from build123d import *

# Parameters (mm, degrees)
F0_W      = 86
F0_H      = 45
F1_DEPTH  = 3
F2_R      = 1.35
F2_W      = 68
F2_H      = 41
F3_DEPTH  = 22
F4_R      = 1.4
F5_DEPTH  = 6
F7_DEPTH  = 3.001
F8_R      = 3
F9_W      = 2
F9_H      = 28
F9_H_2    = 8
F10_DEPTH = 2.5


with BuildPart() as f1:
    # F0 (on Top) → F1 (new body)
    with BuildSketch(Plane.XY):
        Rectangle(F0_W, F0_H)
    extrude(amount=F1_DEPTH)

    # F2 (on face) → F3 (join)
    with BuildSketch(Plane.XY.offset(3)):
        Polygon((43, 22.5), (-43, 22.5), (-43, 14.5), (-36, 14.5), (-36, -14.5), (-43, -14.5), (-43, -22.5), (43, -22.5), (43, -14.5), (36, -14.5), (36, 14.5), (43, 14.5), align=None)
        with Locations((-39, -18.5)):
            Circle(F2_R, mode=Mode.SUBTRACT)
        with Locations((39, -18.5)):
            Circle(F2_R, mode=Mode.SUBTRACT)
        with Locations((-39, 18.5)):
            Circle(F2_R, mode=Mode.SUBTRACT)
        Rectangle(F2_W, F2_H, mode=Mode.SUBTRACT)
        with Locations((39, 18.5)):
            Circle(F2_R, mode=Mode.SUBTRACT)
    extrude(amount=F3_DEPTH)

    # F4 (on face) → F5 (join)
    with BuildSketch(Plane.XY.offset(3)):
        with BuildLine():
            Line((-28.9413119942, 15.2550414599), (-29.2586880058, 15.2550414599))
            ThreePointArc((-29.2586880058, 15.2550414599), (-29.1, 15.25), (-28.9413119942, 15.2550414599))
        make_face()
        with BuildLine():
            Line((-34, 15.2550414599), (-29.2586880058, 15.2550414599))
            Line((-29.2586880058, 15.2550414599), (-28.9413119942, 15.2550414599))
            ThreePointArc((-28.9413119942, 15.2550414599), (-27.3470376902, 15.9675513639), (-26.6080353575, 17.5497196457))
            Line((-26.6080353575, 17.5497196457), (-26.6080353575, 17.9502803543))
            Line((-26.6080353575, 17.9502803543), (-26.6080353575, 20.5))
            Line((-26.6080353575, 20.5), (-34, 20.5))
            Line((-34, 20.5), (-34, 15.2550414599))
        make_face()
        with Locations((-29.1, 17.75)):
            Circle(F4_R, mode=Mode.SUBTRACT)
        with BuildLine():
            Line((-26.6080353575, 17.9502803543), (-26.6080353575, 17.5497196457))
            ThreePointArc((-26.6080353575, 17.5497196457), (-26.6, 17.75), (-26.6080353575, 17.9502803543))
        make_face()
        with BuildLine():
            Line((-26.5361216883, -20.5), (-26.6006603156, -17.6925444326))
            ThreePointArc((-26.6006603156, -17.6925444326), (-27.2968273142, -16.018362548), (-28.9414728026, -15.2550312371))
            Line((-28.9414728026, -15.2550312371), (-29.2585271974, -15.2550312371))
            Line((-29.2585271974, -15.2550312371), (-34, -15.2550312371))
            Line((-34, -15.2550312371), (-34, -20.5))
            Line((-34, -20.5), (-26.5361216883, -20.5))
        make_face()
        with Locations((-29.1, -17.75)):
            Circle(F4_R, mode=Mode.SUBTRACT)
        with BuildLine():
            Line((-29.2585271974, -15.2550312371), (-28.9414728026, -15.2550312371))
            ThreePointArc((-28.9414728026, -15.2550312371), (-29.1, -15.25), (-29.2585271974, -15.2550312371))
        make_face()
        with BuildLine():
            Line((26.6080353575, 17.5497196457), (26.6080353575, 17.9502803543))
            ThreePointArc((26.6080353575, 17.9502803543), (26.6, 17.75), (26.6080353575, 17.5497196457))
        make_face()
        with BuildLine():
            Line((26.6080353575, 20.5), (26.6080353575, 17.9502803543))
            Line((26.6080353575, 17.9502803543), (26.6080353575, 17.5497196457))
            ThreePointArc((26.6080353575, 17.5497196457), (27.4045208473, 15.9127873169), (29.1, 15.25))
            ThreePointArc((29.1, 15.25), (29.1012864239, 15.250000331), (29.1025728475, 15.2500013239))
            Line((29.1025728475, 15.2500013239), (34, 15.2550414599))
            Line((34, 15.2550414599), (34, 20.5))
            Line((34, 20.5), (26.6080353575, 20.5))
        make_face()
        with Locations((29.1, 17.75)):
            Circle(F4_R, mode=Mode.SUBTRACT)
        with BuildLine():
            Line((28.9479452437, -15.2546284142), (29.2524526886, -15.254652694))
            ThreePointArc((29.2524526886, -15.254652694), (29.1001993362, -15.2500000079), (28.9479452437, -15.2546284142))
        make_face()
        with BuildLine():
            Line((34, -15.2550312371), (29.2524526886, -15.254652694))
            Line((29.2524526886, -15.254652694), (28.9479452437, -15.2546284142))
            ThreePointArc((28.9479452437, -15.2546284142), (27.236154388, -16.0838428842), (26.6032541645, -17.8775156186))
            Line((26.6032541645, -17.8775156186), (26.7371915935, -20.5))
            Line((26.7371915935, -20.5), (34, -20.5))
            Line((34, -20.5), (34, -15.2550312371))
        make_face()
        with Locations((29.1, -17.75)):
            Circle(F4_R, mode=Mode.SUBTRACT)
    extrude(amount=F5_DEPTH)

    # F6 (on face) → F7 (cut, through all)
    with BuildSketch(Plane.XY.offset(3)):
        with BuildLine():
            Line((-43, 8.25), (-40, 8.25))
            ThreePointArc((-40, 8.25), (-38.25, 10), (-40, 11.75))
            Line((-40, 11.75), (-43, 11.75))
            Line((-43, 11.75), (-43, 8.25))
        make_face()
        with BuildLine():
            Line((-43, -11.75), (-40, -11.75))
            ThreePointArc((-40, -11.75), (-38.25, -10), (-40, -8.25))
            Line((-40, -8.25), (-43, -8.25))
            Line((-43, -8.25), (-43, -11.75))
        make_face()
        with BuildLine():
            ThreePointArc((40, 11.75), (38.25, 10), (40, 8.25))
            Line((40, 8.25), (43, 8.25))
            Line((43, 8.25), (43, 11.75))
            Line((43, 11.75), (40, 11.75))
        make_face()
        with BuildLine():
            ThreePointArc((40, -8.25), (38.25, -10), (40, -11.75))
            Line((40, -11.75), (43, -11.75))
            Line((43, -11.75), (43, -8.25))
            Line((43, -8.25), (40, -8.25))
        make_face()
    extrude(amount=-F7_DEPTH, mode=Mode.SUBTRACT)

    # F8
    f8_edges = [f1.edges().sort_by_distance(p)[0] for p in [
        (-43, -22.5, 12.5),
        (-43, 14.5, 14),
        (-43, 22.5, 12.5),
        (-43, -14.5, 14),
        (43, -22.5, 12.5),
        (43, -14.5, 14),
        (43, 14.5, 14),
        (43, 22.5, 12.5),
    ]]
    fillet(f8_edges, radius=F8_R)

    # F9 (on face) → F10 (cut)
    with BuildSketch(Plane.XY.offset(25)):
        with Locations((-35, 0)):
            Rectangle(F9_W, F9_H)
        with Locations((35, -9.5)):
            Rectangle(F9_W, F9_H_2)
    extrude(amount=-F10_DEPTH, mode=Mode.SUBTRACT)


solid = f1.part
Work out the finished part from the listing and answer in its coordinate system (mm). A direction names the side the tool comes from. Give positions to 0.01 mm unless a question says otherwise; leave off trailing zeros. Write each loop counter-clockwise with the first axis right and the second up, starting at its lowest first coordinate (ties: lowest second). Pieces come first, ordered by that corner, then holes.
Q1. The part is cut by section C-C on y = 10. Give the vertices of the cut face in (x, z).
Answer:
outline: (-38.25, 0) - (38.25, 0) - (38.25, 3) - (36, 3) - (36, 25) - (34, 25) - (34, 3) - (-34, 3) - (-34, 22.5) - (-36, 22.5) - (-36, 3) - (-38.25, 3) - close
Q2. A tool of negligible diameter and unlimited length cuts with its end or side. For faces 5 (the face through (38, -14.5, 14)), 6 (the face through (35, -5.5, 24)), 7 (the face through (-39.29, 17.18, 13.85)), from which of +Z, -Z, +X, -X, +Y, -Y can it reach the whole face along a straight path? Write none if from no direction.
Answer:
face 5: +Z, +X
face 6: +Z, +X, -X
face 7: +Z
Q3. The part is cut by section A-A on z = 23.75. State how many separate pieces and enclosed holes the cut face has, and give its area (3 significant figures).
Answer:
separate pieces: 2
enclosed holes: 4
area: 566 mm2
Q4. Straight lines are drawn through the part: L1, parallel to Y at x = -29, z = 6.5; L2, parallel to Y at x = 39, z = 8.25; L3, parallel to Y at x = 9, z = 22. For each, find the intervals that lie inside material, in ascending order.
Answer:
L1: y = -22.5 to -19.15, -16.35 to -15.25, 15.25 to 16.35, 19.15 to 22.5
L2: y = -22.5 to -19.85, -17.15 to -14.5, 14.5 to 17.15, 19.85 to 22.5
L3: y = -22.5 to -20.5, 20.5 to 22.5
Q5. The part is cut by section D-D on y = -3. Give the vertices of the cut face in (x, z).
Answer:
outline: (-43, 0) - (43, 0) - (43, 3) - (36, 3) - (36, 25) - (34, 25) - (34, 3) - (-34, 3) - (-34, 22.5) - (-36, 22.5) - (-36, 3) - (-43, 3) - close
Q6. The part is cut by section B-B on x = -19. Give the vertices of the cut face in (y, z).
Answer:
outline: (-22.5, 0) - (22.5, 0) - (22.5, 25) - (20.5, 25) - (20.5, 3) - (-20.5, 3) - (-20.5, 25) - (-22.5, 25) - close
Q7. Given pin 1 (2 mm diameter, centred on y = 3, z = 9, fed in from +X); pin 2 (6.5 mm diameter, centred on y = 6, z = 14.5, fed in from -X); pin 3 (2 mm diameter, centred on x = -6.5, y = -11, fed in from +Z), each flat-ended and moving along its own axis, determine where each tip first touches the part or whether it passes through.
Answer:
pin 1: stops at x = 36
pin 2: stops at x = -36
pin 3: stops at z = 3
Q8. For a pull along Y with two mould halves and no side action, classify faces 1 (the face through (1, 22.5, 12)), 2 (the face through (42, -8.25, 2)), 3 (the face through (43, 0, 1)), 4 (the face through (31, 18, 9)) as released by +Y, released by -Y, zero draft, split by the parting line, or undercut.
Answer:
face 1: released by +Y
face 2: undercut
face 3: zero draft
face 4: undercut
